Read the model definition and answer for the solid it produces. Units are mm, in the model's axes. Give positions to 0.01 mm unless a question says otherwise; leave off trailing zeros. Write each loop counter-clockwise with the first axis right and the second up, starting at its lowest first coordinate (ties: lowest second). Pieces come first, ordered by that corner, then holes. Notation, with made-up numbers: M 63,59 L 92,59 A29 cw 92,81 Z; hole C 86.25,75 d2. An arc over 180 degrees is marked long. Use a Markdown table: item, result. Add a question column.
Item 1: Consider probe 1 along Z at (x, y) = (1.1, 0); probe 2 along X at (y, z) = (2.35, 0); probe 3 along Y at (x, z) = (1.85, 2.5). Determine where each line is inside the solid, lowest interval first. Write a range as [from, to].
Item 2: A cutting plane is placed at C-C on x = 2.25. Determine the outline of the cut face in (y, z).
Item 3: A cutting plane is placed at D-D on x = 0. Determine the outline of the cut face in (y, z).
Item 4: Given P1, Ø1.5, axis at x = 1.5, y = -1.5, coming from the +Z side; P2, Ø3, axis at x = -1.5, y = 2.5, coming from the -Z side; P3, Ø2.5, axis at y = 0, z = 0, coming from the +X side; P4, Ø2, axis at x = 2, z = 1.5, coming from the -Y side, each flat-ended and moving along its own axis, determine where each tip first touches the part or whether it passes through.
Item 5: The mould has two halves that part along Z. Classify faces 1 (the cylindrical face through (0.03, -1.5, 0.07)), 2 (the cylindrical face through (0.747, 2.267, 0.235)), 3 (the cylindrical face through (0.219, 3.233, 1.341)), 4 (the flat face through (-2.5, 1.3, -1.3)): pulls with the +Z half, pulls with the -Z half, needs draft (parallel to the pull), parting line crosses it, or undercut.
Item 6: A cutting plane is placed at B-B on z = 0. Determine the outline of the cut face in (x, y), then the cut area to 3 significant figures.
Item 7: A cutting plane is placed at A-A on y = 0. Determine the outline of the cut face in (x, z).
Autodesk Inventor part; units mm, degrees
ref_plane "gst_nr_1_XY" through (0, 3.5, 0) normal (0, 1, 0) x (1, 0, 0)
ref_plane "gst_nr_1_YZ" through (0, 3.5, 0) normal (1, 0, 0) x (0, 0, -1)
ref_plane "gst_nr_1_ZX" through (0, 3.5, 0) normal (0, 0, -1) x (0, 1, 0)
sketch "Skizze_1" plane through (0, 0, 0) normal (0, 0, 1) x (1, 0, 0)
  line L0 (2.5, 0) -> (-2.5, 0)
  line L1 (-2.5, 3) -> (-2.5, 1.553)
  line L2 (-2.5, 1.553) -> (-2.447, 1.5)
  line L3 (-2.447, 1.5) -> (2.447, 1.5)
  line L4 (2.447, 1.5) -> (2.5, 1.553)
  line L5 (2.5, 1.553) -> (2.5, 3.5)
  line L6 (2.5, 3.5) -> (-2, 3.5)
  line L7 (-2, 3.5) -> (-2.5, 3)
revolve "Revolution1" add sketch "Skizze_1" angle 360 about axis through (2.5, 0, 0) along (1, 0, 0)
sketch "Skizze_2" plane through (0, 0, 0) normal (0, 0, 1) x (1, 0, 0)
  line L0 (0, 0.75) -> (0, 3.5)
  line L1 (0, 3.5) -> (1, 3.5)
  line L2 (1, 3.5) -> (0.7835, 3.2835)
  line L3 (0.7835, 3.2835) -> (0.7835, 0.9665)
  line L4 (0.7835, 0.9665) -> (1, 0.75)
  line L5 (1, 0.75) -> (0, 0.75)
  line L6 (0, 0.75) -> (0, 3.5)
revolve "Revolution2" cut sketch "Skizze_2" angle 360 about axis through (0, 0.75, 0) along (0, -1, 0)
thread "Thread1"
ref_plane "gst_nr_1_XY" through (0, 3.5, 0) normal (0, 1, 0) x (1, 0, 0)
ref_plane "gst_nr_1_YZ" through (0, 3.5, 0) normal (1, 0, 0) x (0, 0, -1)
ref_plane "gst_nr_1_ZX" through (0, 3.5, 0) normal (0, 0, -1) x (0, 1, 0)
properties part number "623890036_1"
Filled in:
| question | item | result |
|---|---|---|
| 1 | probe 1 | [-3.5, -1.5], [1.5, 3.5] |
| 1 | probe 2 | [-2.5, -0.78], [0.78, 2.5] |
| 1 | probe 3 | [-2.45, 2.45] |
| 2 | outline | C 0,0 d7; hole C 0,0 d3 |
| 3 | outline | M 1.28,-0.78 A1.5 cw long 1.28,0.78 L 3.28,0.78 L 3.39,0.89 A3.5 ccw long 3.39,-0.89 L 3.28,-0.78 Z |
| 4 | P1 | z = 3.42 |
| 4 | P2 | z = -3.35 |
| 4 | P3 | through |
| 4 | P4 | y = -3.46 |
| 5 | face 1 | undercut |
| 5 | face 2 | undercut |
| 5 | face 3 | parting line crosses it |
| 5 | face 4 | needs draft |
| 6 | outline | M -2.5,-3 L -2,-3.5 L 2.5,-3.5 L 2.5,-1.55 L 2.45,-1.5 L -2.45,-1.5 L -2.5,-1.55 Z; M -2.5,1.55 L -2.45,1.5 L -0.78,1.5 L -0.78,3.28 L -1,3.5 L -2,3.5 L -2.5,3 Z; M 0.78,1.5 L 2.45,1.5 L 2.5,1.55 L 2.5,3.5 L 1,3.5 L 0.78,3.28 Z |
| 6 | area | 16.6 mm² |
| 7 | outline | M -2.5,-3 L -2,-3.5 L 2.5,-3.5 L 2.5,-1.55 L 2.45,-1.5 L -2.45,-1.5 L -2.5,-1.55 Z; M -2.5,1.55 L -2.45,1.5 L 2.45,1.5 L 2.5,1.55 L 2.5,3.5 L -2,3.5 L -2.5,3 Z |
